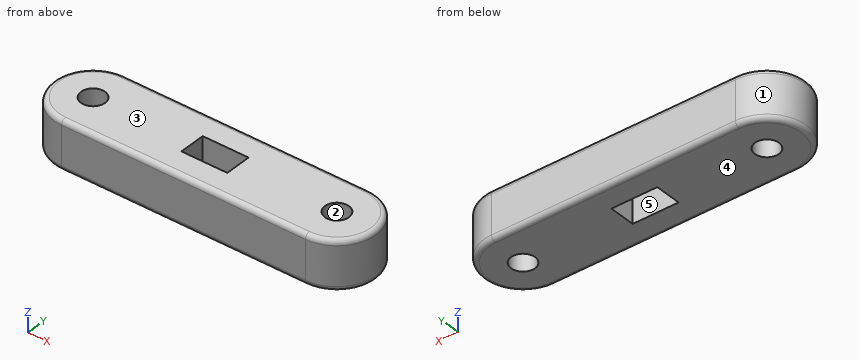
Solid Edge part; units mm, degrees
sketch "Sketch1" plane through (0, 0, 0) normal (0, 0, 1) x (1, 0, 0)
  line L0 (-2.35, -1.35) -> (2.35, -1.35)
  line L1 (2.35, -1.35) -> (2.35, 1.35)
  line L2 (2.35, 1.35) -> (-2.35, 1.35)
  line L3 (-2.35, 1.35) -> (-2.35, -1.35)
  line L4 (12.5, 4) -> (-12.5, 4)
  line L5 (-12.5, -4) -> (12.5, -4)
  arc A0 (-12.5, -4) -> (-12.5, 4) centre (-12.5, 0) cw
  arc A1 (12.5, 4) -> (12.5, -4) centre (12.5, 0) cw
extrude "Protrusion1" add sketch "Sketch1" along normal blind 5
fillet "Round_1" radius 0.5 6 edges at (0, 4, 5) (-16.5, 0, 5) (16.5, 0, 5) (0, -4, 0) (16.5, 0, 0) (-16.5, 0, 0)
hole "Hole_3" at (12.5, 0, 5) direction (0, 0, -1) diameter 2.459 end through all
hole "Hole1" at (-12.5, 0, 5) direction (0, 0, -1) diameter 2.459 end through all
Here's how the part is built. I have some questions about the finished solid (model axes, mm). Face numbers are marked on the shaded views. A direction names the side the tool comes from. Round coordinates to 2 decimals unless told otherwise and drop trailing zeros. Order: outer loops, then holes, each group sorted by start corner. A loop starts at its lowest first (then second) coordinate and runs counter-clockwise, first axis right, second up. Notation, with made-up numbers: (2, -1) -> (53, -1) arc R22 ccw to (53, 29) -> close; hole circle Ø9 at (-19, 6). An arc over 180 degrees is marked (long way). Use CSV: the item, a comma, the result in double quotes.
1. I want a section at A-A on x = -0.5. List the corners of the cut face in (y, z) for me.
Recorded:
outline,"(-4, 0.5) arc R0.5 ccw to (-3.5, 0) -> (-1.35, 0) -> (-1.35, 5) -> (-3.5, 5) arc R0.5 ccw to (-4, 4.5) -> close; (1.35, 0) -> (3.5, 0) arc R0.5 ccw to (4, 0.5) -> (4, 4.5) arc R0.5 ccw to (3.5, 5) -> (1.35, 5) -> close"
2. I want a section at C-C on z = 1.7. List the corners of the cut face in (x, y) for me, and give its area (3 significant figures).
Recorded:
outline,"(-12.5, -4) -> (12.5, -4) arc R4 ccw to (12.5, 4) -> (-12.5, 4) arc R4 ccw to start; hole circle Ø2.46 at (-12.5, 0); hole (-2.35, -1.35) -> (2.35, -1.35) -> (2.35, 1.35) -> (-2.35, 1.35) -> close; hole circle Ø2.46 at (12.5, 0)"
area,"228 mm2"
3. I need wall thicknesses on line 1 along X through (y, z) = (0, 2.2); line 2 along Y through (x, z) = (1, 2.9); line 3 along Y through (x, z) = (12.5, 2.8). Which ranges of each line are inside material? Lowest first, please.
Recorded:
line 1,"x = -16.5 to -13.73, -11.27 to -2.35, 2.35 to 11.27, 13.73 to 16.5"
line 2,"y = -4 to -1.35, 1.35 to 4"
line 3,"y = -4 to -1.23, 1.23 to 4"
4. I'm going to push flat-ended pins straight in: P1, Ø2, axis at y = -0.5, z = 3, coming from the +X side; P2, Ø2, axis at y = 3, z = 1, coming from the +X side. Where does each tip first touch, or does it pass through?
Recorded:
P1,"stops at x = 16.5"
P2,"stops at x = 15.96"
5. Thinking about a two-plate mould opening in X: for the marked faces 1, 2 and 3, which applies, pulls with the +X half, pulls with the -X half, needs draft (parallel to the pull), parting line crosses it, or undercut?
Recorded:
face 1,"pulls with the -X half"
face 2,"undercut"
face 3,"needs draft"
6. I want a section at B-B on y = 0. List the corners of the cut face in (x, z) for me.
Recorded:
outline,"(-16.5, 0.5) arc R0.5 ccw to (-16, 0) -> (-13.73, 0) -> (-13.73, 5) -> (-16, 5) arc R0.5 ccw to (-16.5, 4.5) -> close; (-11.27, 0) -> (-2.35, 0) -> (-2.35, 5) -> (-11.27, 5) -> close; (2.35, 0) -> (11.27, 0) -> (11.27, 5) -> (2.35, 5) -> close; (13.73, 0) -> (16, 0) arc R0.5 ccw to (16.5, 0.5) -> (16.5, 4.5) arc R0.5 ccw to (16, 5) -> (13.73, 5) -> close"
7. Which directions (+Z, -Z, +X, -X, +Y, -Y) give clear straight access to the entire face, cutting with the end or side of a thin tool? Please do the marked faces 4 and 5.
Recorded:
face 4,"-Z, +X, -X, +Y, -Y"
face 5,"+Z, -Z"
